Autodesk Inventor part; units mm, degrees
ref_plane "YZ Plane" through (0, 0, 0) normal (1, 0, 0) x (0, 1, 0)
ref_plane "XZ Plane" through (0, 0, 0) normal (0, 1, 0) x (-1, 0, 0)
ref_plane "XY Plane" through (0, 0, 0) normal (0, 0, 1) x (1, 0, 0)
sketch "Эскиз1" plane through (0, 0, 0) normal (0, 0, 1) x (1, 0, 0)
  line L0 (29.925, -19.7625) -> (39.925, -19.7625)
  line L1 (39.925, -19.7625) -> (39.925, -34.7625)
  line L2 (39.925, -34.7625) -> (29.925, -34.7625)
  line L3 (29.925, -34.7625) -> (29.925, -19.7625)
  point P0 (0, 0)
  dimension "d0" = 15
  dimension "d1" = 10
extrude "Выдавливание1" add sketch "Эскиз1" along normal blind 5
sketch "Эскиз2" plane through (29.925, -34.7625, 0) normal (0, -1, 0) x (1, 0, 0)
  line L0 (0, 0) -> (0, 5)
  line L1 (0, 1) -> (4.25, 1)
  line L2 (4.25, 1) -> (4.25, 4)
  line L3 (4.25, 4) -> (5.75, 4)
  line L4 (5.75, 4) -> (5.75, 1)
  line L5 (5.75, 1) -> (10, 1)
  line L6 (10, 0) -> (10, 5)
  line L7 (0, 5) -> (10, 5)
  line L8 (0, 0) -> (10, 0)
  point P0 (-29.925, 0)
  dimension "d4" = 1.5
  dimension "d5" = 4.25
  dimension "d6" = 10
  dimension "d7" = 1
  dimension "d8" = 1
extrude "Выдавливание2" cut sketch "Эскиз2" against normal through all contours L0 L1 L2 L3 L4 L5 L6 L8 keep common part
sketch "Эскиз3" plane through (35.675, -34.7625, 4) normal (1, 0, 0) x (0, 0, -1)
  line L0 (3, 15) -> (0, 15)
  line L1 (0, 0) -> (0, 15)
  line L2 (0, 0) -> (3, 0)
  line L3 (3, 0) -> (3, 15)
  line L4 (3, 0) -> (3, 15)
  line L5 (3, 1) -> (1, 1)
  line L6 (1, 1) -> (1, 14)
  line L7 (1, 14) -> (3, 14)
  line L8 (3, 14) -> (3, 1)
  point P0 (4, 34.7625)
  point P1 (3, 1)
  dimension "d11" = 1
  dimension "d12" = 1
  dimension "d13" = 1
extrude "Выдавливание3" cut sketch "Эскиз3" against normal through all contours L3 L5 L6 L7
equation "\"d5\" = -0.5 * d4 + 0.5 * d6"
properties part number "Клемники винтовые"
The listing builds one solid part. Answer for the finished solid, in the listing's coordinates (mm). A direction names the side the tool comes from. Round coordinates to 2 decimals unless told otherwise and drop trailing zeros. Order: outer loops, then holes, each group sorted by start corner. A loop starts at its lowest first (then second) coordinate and runs counter-clockwise, first axis right, second up. Notation, with made-up numbers: M 35.5,-25 L 62.5,-25 A20 cw 62.5,-9 Z; hole C 24,72.25 d11. An arc over 180 degrees is marked long. Answer in a Markdown table with one row per item. Add a question column.
1) The part is cut by section A-A on z = 2.4. Determine the outline of the cut face in (x, y) (1 decimal).
2) Which of the six approach directions +Z, -Z, +X, -X, +Y, -Y give full straight-line access (tool end or side, diameter ignored) to faces 5 (the face through (34.175, -27.4, 3.5)), 6 (the face through (39.925, -27.2, 0.5)), 7 (the face through (35, -27, 3)), 8 (the face through (35.675, -27.4, 3.2))?
3) The part is cut by section B-B on x = 35.25. Determine the outline of the cut face in (y, z), plus the area to 3 significant figures.
4) The part is cut by section D-D on x = 33. Determine the outline of the cut face in (y, z), plus the area to 3 significant figures.
5) Determine the mould class of faces 1 (the face through (35, -27, 0)), 2 (the face through (35, -20.762, 2)), 3 (the face through (35, -27, 4)), 4 (the face through (29.925, -27.4, 0.5)) for opening direction Z: pulls with the +Z half, pulls with the -Z half, needs draft (parallel to the pull), parting line crosses it, or undercut.
6) The part is cut by section C-C on y = -28.75. Determine the outline of the cut face in (x, z) (3 decimals).
7) Consider line 1 along Z through (x, y) = (34.75, -29.5); line 2 along Z through (x, y) = (37, -25.5); line 3 along X through (y, z) = (-27.5, 3.35) (3 decimals). Determine where each line is inside the solid, lowest interval first. Write a range as from..to.
8) A flat-ended cylindrical pin translates along its axis: pin 1 Ø1.5 at (y, z) = (-29.5, 3) entering from -X (3 decimals). Find the tip coordinate at first contact, or state that the pin passes through.
Findings below:
| question | item | result |
|---|---|---|
| 1 | outline | M 34.2,-34.8 L 35.7,-34.8 L 35.7,-33.8 L 34.2,-33.8 Z; M 34.2,-20.8 L 35.7,-20.8 L 35.7,-19.8 L 34.2,-19.8 Z |
| 2 | face 5 | +Z, -X, +Y, -Y |
| 2 | face 6 | +Z, -Z, +X, +Y, -Y |
| 2 | face 7 | +X, -X |
| 2 | face 8 | +Z, +X, +Y, -Y |
| 3 | outline | M -34.76,0 L -19.76,0 L -19.76,4 L -34.76,4 Z; hole M -33.76,1 L -20.76,1 L -20.76,3 L -33.76,3 Z |
| 3 | area | 34.0 mm² |
| 4 | outline | M -34.76,0 L -19.76,0 L -19.76,1 L -34.76,1 Z |
| 4 | area | 15.0 mm² |
| 5 | face 1 | pulls with the -Z half |
| 5 | face 2 | undercut |
| 5 | face 3 | pulls with the +Z half |
| 5 | face 4 | needs draft |
| 6 | outline | M 29.925,0 L 39.925,0 L 39.925,1 L 29.925,1 Z; M 34.175,3 L 35.675,3 L 35.675,4 L 34.175,4 Z |
| 7 | line 1 | z = 0..1, 3..4 |
| 7 | line 2 | z = 0..1 |
| 7 | line 3 | x = 34.175..35.675 |
| 8 | pin 1 | stops at x = 34.175 |
